from build123d import *

# Parameters (mm, degrees)
SKETCH_1_W                     = 130
SKETCH_1_H                     = 347
EXTRUDE_1_DEPTH                = 6
EXTRUDE_2_DEPTH                = 2.5
SKETCH_3_W                     = 65
SKETCH_3_H                     = 65
CUT_EXTRUDE_1_DEPTH            = 371.600863592
EXTRUDE_3_DEPTH                = 2.5
EXTRUDE_4_DEPTH                = 2.5
HOLE_WIZARD_10_0_10_1_D        = 10
HOLE_WIZARD_4_8_4_8_1_D        = 4.8
HOLE_WIZARD_1_D                = 5
HOLE_WIZARD_1_DEPTH            = 8.5
HOLE_WIZARD_1_CBORE_D          = 7.2
HOLE_WIZARD_1_CBORE_DEPTH      = 4
FILLET_1_R                     = 10
SKETCH_14_W                    = 130
SKETCH_14_H                    = 6
EXTRUDE_5_DEPTH                = 25
HOLE_WIZARD_M2_5_1_D           = 3
HOLE_WIZARD_M2_5_1_CBORE_D     = 4.6
HOLE_WIZARD_M2_5_1_CBORE_DEPTH = 3.5
FILLET_2_R                     = 10


with BuildPart() as part:
    # 草图1 → 凸台-拉伸1 (new body)
    with BuildSketch(Plane(origin=(0, 0, 0), x_dir=(-1, 0, 0), z_dir=(0, 0, -1))):
        with Locations((-65, -173.5)):
            Rectangle(SKETCH_1_W, SKETCH_1_H)
    extrude(amount=-EXTRUDE_1_DEPTH)

    # 草图2 → 凸台-拉伸2 (add)
    with BuildSketch(Plane.XY.offset(6)):
        with BuildLine():
            Line((15, -298.5), (115, -298.5))
            ThreePointArc((115, -298.5), (107.915907861, -314.190105481), (97.5, -327.896769368))
            add(Edge.make_bspline(
                [(32.5, -327.896769368), (55.796929517, -351.885684413), (72.679914197, -353.454082804), (97.5, -327.896769368)],
                knots=[0, 0, 0, 0, 1, 1, 1, 1], degree=3))
            ThreePointArc((32.5, -327.896769368), (22.092962751, -314.184824775), (15, -298.5))
        make_face()
    extrude(amount=EXTRUDE_2_DEPTH)

    # 草图3 → 切除-拉伸1 (cut, through all)
    with BuildSketch(Plane.XY.offset(6)):
        with Locations((65, -32.5)):
            Rectangle(SKETCH_3_W, SKETCH_3_H)
    extrude(amount=-CUT_EXTRUDE_1_DEPTH, mode=Mode.SUBTRACT)

    # 草图4 → 凸台-拉伸3 (add)
    with BuildSketch(Plane.XY.offset(6)):
        with BuildLine():
            Line((115, -49), (97.5, -49))
            Line((97.5, -49), (97.5, -19.603230632))
            ThreePointArc((97.5, -19.603230632), (107.915907861, -33.309894519), (115, -49))
        make_face()
    extrude(amount=EXTRUDE_3_DEPTH)

    # 草图5 → 凸台-拉伸4 (add)
    with BuildSketch(Plane.XY.offset(6)):
        with BuildLine():
            Line((32.5, -19.603230632), (32.5, -49))
            Line((32.5, -49), (15, -49))
            ThreePointArc((15, -49), (22.092962751, -33.315175225), (32.5, -19.603230632))
        make_face()
    extrude(amount=EXTRUDE_4_DEPTH)

    # Ø10.0 (10) 直径孔1 (through all)
    with Locations(Plane.XY.offset(6)):
        with Locations((15, -32.5), (115, -32.5)):
            Hole(HOLE_WIZARD_10_0_10_1_D / 2)

    # Ø4.8 (4.8) 直径孔1 (through all)
    with Locations(Plane.XY.offset(6)):
        with Locations((100, -75), (30, -145), (100, -145), (30, -75)):
            Hole(HOLE_WIZARD_4_8_4_8_1_D / 2)

    # 孔1
    with Locations(Plane(origin=(0, 0, 0), x_dir=(-1, 0, 0), z_dir=(0, 0, -1))):
        with Locations((-18, -75), (-112, -210), (-112, -140), (-112, -107.5), (-18, -107.5), (-18, -140), (-18, -210), (-18, -242.5), (-18, -275), (-112, -275), (-112, -242.5), (-112, -75)):
            CounterBoreHole(HOLE_WIZARD_1_D / 2, HOLE_WIZARD_1_CBORE_D / 2, HOLE_WIZARD_1_CBORE_DEPTH, depth=HOLE_WIZARD_1_DEPTH)

    # 圆角1
    fillet_1_edges = [part.edges().sort_by_distance(p)[0] for p in [
        (97.5, 0, 3),
        (32.5, 0, 3),
        (130, 0, 3),
        (0, 0, 3),
    ]]
    fillet(fillet_1_edges, radius=FILLET_1_R)

    # 草图14 → 凸台-拉伸5 (add)
    with BuildSketch(Plane.XZ.offset(347)):
        with Locations((65, 3)):
            Rectangle(SKETCH_14_W, SKETCH_14_H)
    extrude(amount=EXTRUDE_5_DEPTH)

    # M2.5 六角头机械螺钉的柱形沉头孔1 (through all)
    with Locations(Plane.XY.offset(6)):
        with Locations((110.5, -288.5), (19.5, -288.5), (19.5, -367), (110.5, -367)):
            CounterBoreHole(HOLE_WIZARD_M2_5_1_D / 2, HOLE_WIZARD_M2_5_1_CBORE_D / 2, HOLE_WIZARD_M2_5_1_CBORE_DEPTH)

    # 圆角2
    fillet_2_edges = [part.edges().sort_by_distance(p)[0] for p in [
        (0, -372, 3),
        (130, -372, 3),
    ]]
    fillet(fillet_2_edges, radius=FILLET_2_R)


solid = part.part
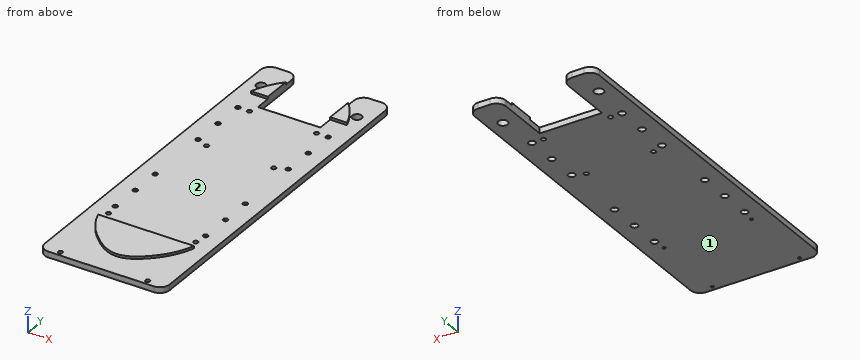
Design review of the part built by this model. Coordinates are the model's own, in mm. Face numbers are marked on the shaded views. Round coordinates to 2 decimals unless told otherwise and drop trailing zeros. Order: outer loops, then holes, each group sorted by start corner. A loop starts at its lowest first (then second) coordinate and runs counter-clockwise, first axis right, second up.
1) For L1, parallel to X at y = -242.5, z = 5.5; L2, parallel to X at y = -288.5, z = 4.8; L3, parallel to Y at x = 100, z = 2, list the stretches that pass through material, from the lowest coordinate up.
The answers:
L1: x = 0 to 15.5, 20.5 to 109.5, 114.5 to 130
L2: x = 0 to 17.2, 21.8 to 108.2, 112.8 to 130
L3: y = -372 to -147.4, -142.6 to -77.4, -72.6 to -3.39
2) Consider section B-B (y = -117.5). State the section outline as (x, z) points, plus the area to 3 significant figures.
The answers:
outline: (0, 0) - (130, 0) - (130, 6) - (0, 6) - close
area: 780 mm2
3) Consider section A-A (y = -311.5). State the section outline as (x, z) points.
The answers:
outline: (0, 0) - (130, 0) - (130, 6) - (109.44, 6) - (109.44, 8.5) - (20.57, 8.5) - (20.57, 6) - (0, 6) - close
4) Draft analysis for pull direction Y (two halves, no side actions). For the marked faces 1 and 2, state which applies: released by +Y, released by -Y, zero draft, split by the parting line, or undercut.
The answers:
face 1: zero draft
face 2: undercut
5) Clearance check with flat-ended pins moving along their axes: pin 1 Ø6 at (x, y) = (18, -210) entering from +Z; pin 2 Ø1 at (x, z) = (23.5, 7) entering from +Y; pin 3 Ø4 at (x, y) = (30, -75) entering from +Z; pin 4 Ø4 at (x, z) = (37.5, 3) entering from +Y. State where each tip first meets the part, or that it passes through.
The answers:
pin 1: stops at z = 6
pin 2: stops at y = -30.28
pin 3: passes through
pin 4: stops at y = -65
